Geometry: final body of the model. Coordinates: model frame, mm. Face numbers are marked on the shaded views. A direction names the side the tool comes from. Give positions to 0.01 mm unless a question says otherwise; leave off trailing zeros. Write each loop counter-clockwise with the first axis right and the second up, starting at its lowest first coordinate (ties: lowest second). Pieces come first, ordered by that corner, then holes.
Q1. Cut plane D-D on z = 43. Return the cut outline in (x, y).
Q2. Reachability of the marked faces 5, 6 and 7 from +Z, -Z, +X, -X, +Y, -Y: full face, straight path, thin tool, end or side. Return the list, or none.
Q3. Line query: L1, parallel to Z at x = -41.5, y = -28.5; L2, parallel to Z at x = 48, y = -28; L3, parallel to Z at x = -0.5, y = -16. Output: solid intervals per line, ascending.
Q4. Cut plane A-A on x = 43.5. Return the cut outline in (y, z).
Q5. Cut plane C-C on y = 18.5. Return the cut outline in (x, z), plus the area to 3 significant figures.
Q6. Cut plane B-B on z = 7.5. Return the cut outline in (x, y), plus the area to 3 significant figures.
Q7. Draft query along Z for the marked faces 1, 2, 3 and 4. Return one class per face: pulls with the +Z half, pulls with the -Z half, needs draft (parallel to the pull), parting line crosses it, or undercut.
Q8. Pin query (flat end, axial travel): pin 1 (23 mm diameter, centred on x = -11.5, y = 11.5, fed in from -Z). Return the tip coordinate at first contact, or that it passes through.
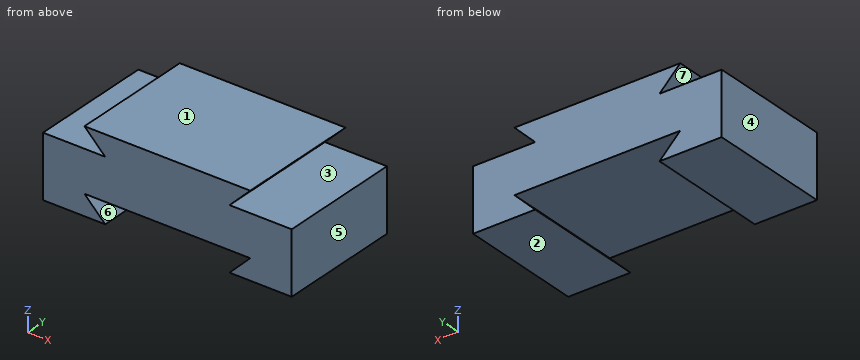
```python
from build123d import *

# Parameters (mm, degrees)
F1_DEPTH = 38.1


with BuildPart() as f1:
    # F0 (on Front) → F1 (new body, symmetric)
    with BuildSketch(Plane.XZ):
        Polygon((0, 50.8), (0, 12.7), (50.8, 12.7), (38.1, 0), (76.2, 0), (76.2, 38.1), (38.1, 38.1), (50.8, 50.8), align=None)
    extrude(amount=F1_DEPTH, both=True)

    # F2: F1 across face


with BuildPart() as f1_1:
    add(f1.part)
    add(f1.part.mirror(Plane(origin=(0, 0, 31.75), x_dir=(0, -1, 0), z_dir=(-1, 0, 0))))


solid = f1_1.part
```
Data:
1. outline: (-43, -38.1) - (43, -38.1) - (43, 38.1) - (-43, 38.1) - close
2. face 5: +Z, -Z, +X, +Y, -Y
2. face 6: +Y, -Y
2. face 7: -X, +Y, -Y
3. L1: z = 0 to 3.4, 12.7 to 38.1, 41.5 to 50.8
3. L2: z = 0 to 9.9, 12.7 to 38.1, 48 to 50.8
3. L3: z = 12.7 to 50.8
4. outline: (-38.1, 0) - (38.1, 0) - (38.1, 5.4) - (-38.1, 5.4) - close; (-38.1, 12.7) - (38.1, 12.7) - (38.1, 38.1) - (-38.1, 38.1) - close; (-38.1, 43.5) - (38.1, 43.5) - (38.1, 50.8) - (-38.1, 50.8) - close
5. outline: (-76.2, 0) - (-38.1, 0) - (-50.8, 12.7) - (50.8, 12.7) - (38.1, 0) - (76.2, 0) - (76.2, 38.1) - (38.1, 38.1) - (50.8, 50.8) - (-50.8, 50.8) - (-38.1, 38.1) - (-76.2, 38.1) - close
5. area: 5,810 mm2
6. outline: (-76.2, -38.1) - (-45.6, -38.1) - (-45.6, 38.1) - (-76.2, 38.1) - close; (45.6, -38.1) - (76.2, -38.1) - (76.2, 38.1) - (45.6, 38.1) - close
6. area: 4,660 mm2
7. face 1: pulls with the +Z half
7. face 2: pulls with the -Z half
7. face 3: undercut
7. face 4: needs draft
8. pin 1: stops at z = 12.7
